Build history of the part. All positions in model axes, mm. A direction names the side the tool comes from. Round coordinates to 2 decimals unless told otherwise and drop trailing zeros. Order: outer loops, then holes, each group sorted by start corner. A loop starts at its lowest first (then second) coordinate and runs counter-clockwise, first axis right, second up. Notation, with made-up numbers: (69.5, 45) -> (109.5, 45) arc R34 cw to (109.5, 76) -> close; hole circle Ø5 at (-10, 9). An arc over 180 degrees is marked (long way). Answer as CSV lines item,"result". Start each with the question number.
```python
from build123d import *

# Parameters (mm, degrees)
ESQUISSE1_R             = 6.3
BOSS_EXTRU_1_DEPTH      = 5
ESQUISSE4_W             = 5
ESQUISSE4_H             = 25
ESQUISSE4_H_2           = 10
BOSS_EXTRU_2_DEPTH      = 5
ENL_V_MAT_EXTRU_1_DEPTH = 5


with BuildPart() as part:
    # Esquisse1 → Boss.-Extru.1 (new body)
    with BuildSketch(Plane.XY):
        Polygon((-65, 51.461253746), (0, 40), (0, -40), (-65, -51.461253746), (-65, -71.461253746), (-20.625899742, -71.461253746), (25, -63.416176602), (25, 63.800831685), (-18.444412366, 71.461253746), (-65, 71.461253746), align=None)
        with Locations((-20, 53.680805733)):
            Circle(ESQUISSE1_R, mode=Mode.SUBTRACT)
        with Locations(Location((10, -5, 0), (0, 0, 180))):
            Circle(ESQUISSE1_R, mode=Mode.SUBTRACT)
    extrude(amount=BOSS_EXTRU_1_DEPTH)

    # Esquisse4 → Boss.-Extru.2 (add)
    with BuildSketch(Plane.XY.offset(5)):
        with Locations((-2.5, -7.5)):
            Rectangle(ESQUISSE4_W, ESQUISSE4_H)
        Polygon((-11.888404247, 42.096246426), (-31.584559307, 45.56920998), (-32.452800195, 40.645171215), (-12.756645135, 37.172207661), align=None)
        Polygon((-9.84807753, -41.736481777), (-24.620193825, -44.341204442), (-25.488434714, -39.417165677), (-10.716318418, -36.812443012), align=None)
        with Locations((-2.5, 25)):
            Rectangle(ESQUISSE4_W, ESQUISSE4_H_2)
        Polygon((-54.164426416, -49.550649772), (-39.39231012, -46.945927107), (-40.260551009, -42.021888342), (-55.032667304, -44.626611007), align=None)
        Polygon((-44.316348886, 47.814167995), (-54.164426416, 49.550649772), (-55.032667304, 44.626611007), (-45.184589774, 42.89012923), align=None)
    extrude(amount=-BOSS_EXTRU_2_DEPTH)

    # Esquisse5 → Enlèv. mat.-Extru.1 (cut)
    with BuildSketch(Plane.XY.offset(5)):
        Polygon((-65, 70.461253746), (-18.53190103, 70.461253746), (24, 62.961732054), (24, -62.577076971), (-20.713388405, -70.461253746), (-65, -70.461253746), (-65, -77.148207451), (34.423224657, -77.148207451), (34.423224657, 88.893594993), (-65, 88.893594993), align=None)
    extrude(amount=-ENL_V_MAT_EXTRU_1_DEPTH, mode=Mode.SUBTRACT)


solid = part.part
```
Q1. Slice it at B-B, the plane y = -23. Write the cut outline in (x, z), plus the area to 3 significant figures.
Q2. Slice it at D-D, the plane y = 21.5. Write the cut outline in (x, z), plus the area to 3 significant figures.
Q3. Two-plate mould, pull along Y, no slides. Class faces 4 (the face through (-59.66, 50.52, 2.46)), 5 (the face through (-42, 70.461, 3)), 6 (the face through (-3, 30, 3)): +Y half, -Y half, draft (parallel to the pull), parting line (faces both ways), or undercut.
Q4. Slice it at A-A, the plane x = 11. Write the cut outline in (y, z).
Q5. Slice it at C-C, the plane z = 0.8. Count the separate pieces of the cut face and the enclosed holes in it, plus the area to 3 significant figures.
Q6. Flat gauge pins, fed straight in: pin 1 Ø2.5 at (y, z) = (12, 3) entering from -X; pin 2 Ø2.5 at (x, z) = (-2, 2) entering from +Y; pin 3 Ø1.5 at (y, z) = (-8, 3.5) entering from -X. Where does each tip first touch, or does it go through?
Q7. Probe L1, parallel to Y at x = -2.5, z = 0.3; L2, parallel to Y at x = -20, z = 3.5; L3, parallel to X at y = 8.5, z = 4. List the from-to ranges inside material, lowest first.
Q8. Which spindle directions (+Z, -Z, +X, -X, +Y, -Y) get a long thin tool onto all of the face, cutting with end or side? Do faces 1 (the face through (-32.013, 43.142, 2.535)), 2 (the face through (-59.506, -50.493, 2.465)), 3 (the face through (2.436, 66.764, 2.535)). Say none if no direction does.
Solutions:
1,outline,"(0, 0) -> (24, 0) -> (24, 5) -> (0, 5) -> close"
1,area,"120 mm2"
2,outline,"(-5, 0) -> (24, 0) -> (24, 5) -> (-5, 5) -> close"
2,area,"145 mm2"
3,face 4,"undercut"
3,face 5,"+Y half"
3,face 6,"undercut"
4,outline,"(-64.87, 0) -> (-11.22, 0) -> (-11.22, 5) -> (-64.87, 5) -> close; (1.22, 0) -> (65.25, 0) -> (65.25, 5) -> (1.22, 5) -> close"
5,separate pieces,"1"
5,enclosed holes,"2"
5,area,"6,490 mm2"
6,pin 1,"stops at x = 0"
6,pin 2,"stops at y = 67.77"
6,pin 3,"stops at x = -5"
7,L1,"y = -67.25 to -40.44, -20 to 5, 20 to 30, 40.44 to 67.63"
7,L2,"y = -70.34 to -38.45, 38.45 to 47.38, 59.98 to 70.46"
7,L3,"x = 0 to 24"
8,face 1,"+Z, -Z"
8,face 2,"+Z, -Z, -X"
8,face 3,"+Z, -Z, +X, +Y"
